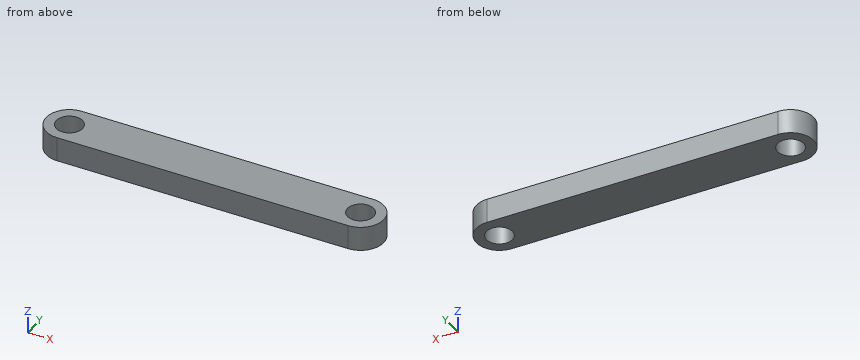
from build123d import *

# Parameters (mm, degrees)
PAD_DEPTH   = 3.175
SKETCH001_R = 1.7
HOLE_DEPTH  = 3.176


with BuildPart() as part:
    # Sketch → Pad (new body)
    with BuildSketch(Plane.XY):
        with BuildLine():
            ThreePointArc((0, 3), (-3, 0), (0, -3))
            Line((0, -3), (37.5, -3))
            ThreePointArc((37.5, -3), (40.5, 0), (37.5, 3))
            Line((0, 3), (37.5, 3))
        make_face()
    extrude(amount=PAD_DEPTH)

    # Sketch001 (on Face6 of Pad) → Hole (cut, through all)
    with BuildSketch(Plane.XY.offset(3.175)):
        Circle(SKETCH001_R)
        with Locations((37.5, 0)):
            Circle(SKETCH001_R)
    extrude(amount=-HOLE_DEPTH, mode=Mode.SUBTRACT)


solid = part.part
Could you check a few things on this model? Use its own coordinates, in mm. Coordinates: 2 decimals unless noted, no trailing zeros. Loops run counter-clockwise (first coordinate to the right, second up) from the corner with the lowest first, then second, coordinate; pieces in that order, holes last.
1. For P1, Ø1.5, axis at y = -1, z = 2.5, coming from the +X side, with a flat end and sliding along its axis, tell me the tip position at first contact or that it passes through.
2. Imagine slicing it at B-B (z = 1.25). Please give me the cut outline in (x, y).
3. Imagine slicing it at C-C (y = 2.4). Please give me the cut outline in (x, z) (3 decimals).
4. Imagine slicing it at A-A (y = 0). Please give me the cut outline in (x, z) (3 decimals), and give its area (3 significant figures).
5. I need wall thicknesses on L1, parallel to Y at x = 37.5, z = 1.05; L2, parallel to X at y = 0.45, z = 0.5; L3, parallel to X at y = -0.95, z = 1.35. Which ranges of each line are inside material? Lowest first, please.
Computed values:
1. P1: stops at x = 40.49
2. outline: (0, -3) - (37.5, -3) arc R3 ccw to (37.5, 3) - (0, 3) arc R3 ccw to start; hole circle Ø3.4 at (0, 0); hole circle Ø3.4 at (37.5, 0)
3. outline: (-1.8, 0) - (39.3, 0) - (39.3, 3.175) - (-1.8, 3.175) - close
4. outline: (-3, 0) - (-1.7, 0) - (-1.7, 3.175) - (-3, 3.175) - close; (1.7, 0) - (35.8, 0) - (35.8, 3.175) - (1.7, 3.175) - close; (39.2, 0) - (40.5, 0) - (40.5, 3.175) - (39.2, 3.175) - close
4. area: 117 mm2
5. L1: y = -3 to -1.7, 1.7 to 3
5. L2: x = -2.97 to -1.64, 1.64 to 35.86, 39.14 to 40.47
5. L3: x = -2.85 to -1.41, 1.41 to 36.09, 38.91 to 40.35
